Can you work these out from the model? Positions are in its coordinate system, mm. Coordinates: 2 decimals unless noted, no trailing zeros. Order: outer loops, then holes, each group sorted by start corner. A loop starts at its lowest first (then second) coordinate and runs counter-clockwise, first axis right, second up. Notation, with made-up numbers: M -25,65.25 L 28,65.25 A26 ccw 28,85.25 Z; hole C 21,84 d11. An arc over 180 degrees is marked long. Answer as CSV lines item,"result". Start each with the question number.
1. I need wall thicknesses on line 1 along X through (y, z) = (-0.8, 1.25); line 2 along X through (y, z) = (-2.2, 5); line 3 along Z through (x, y) = (10, -1.6). Which ranges of each line are inside material? Lowest first, please. Write a range as from..to.
2. If we mould it in two halves opening along X, with no side actions, what happens to faces 1 (the face through (-11.633, -1.61, 3.643)), 2 (the face through (0, 0, 3)), 3 (the face through (-14.057, -1.61, 3.131)), 4 (the face through (11.666, -1.61, 3.456))? For each: released by +X, released by -X, zero draft, split by the parting line, or undercut.
3. If we section it at D-D (y = -0.5): List the corners of the cut face in (x, z) for me (3 decimals), plus the area to 3 significant figures.
4. If we section it at B-B (y = -2.6): List the corners of the cut face in (x, z) for me (3 decimals).
5. If we section it at A-A (z = 4): List the corners of the cut face in (x, y) for me (3 decimals), plus the area to 3 significant figures.
6. If we section it at C-C (z = 2.5): List the corners of the cut face in (x, y) for me (3 decimals), plus the area to 3 significant figures.
```python
from build123d import *

# Parameters (mm, degrees)
BOSS_EXTRUDE1_DEPTH = 6.35
SKETCH2_R           = 2.159
CUT_EXTRUDE1_DEPTH  = 5.08


with BuildPart() as part:
    # Sketch1 → Boss-Extrude1 (new body)
    with BuildSketch(Plane.XY):
        Polygon((-14.986, 0), (14.986, 0), (13.152912895, -3.175), (-13.152912895, -3.175), align=None)
    extrude(amount=BOSS_EXTRUDE1_DEPTH)

    # Sketch2 → Cut-Extrude1 (cut)
    with BuildSketch(Plane.XZ.offset(3.175)):
        with Locations(Location((-9.525, 3.175, 0), (0, 0, 270))):
            Circle(SKETCH2_R)
        with Locations(Location((9.525, 3.175, 0), (0, 0, 270))):
            Circle(SKETCH2_R)
    extrude(amount=-CUT_EXTRUDE1_DEPTH, mode=Mode.SUBTRACT)


solid = part.part
```
Solved:
1,line 1,"-14.52..-10.5, -8.55..8.55, 10.5..14.52"
1,line 2,"-13.72..-10.68, -8.37..8.37, 10.68..13.72"
1,line 3,"0..1.07, 5.28..6.35"
2,face 1,"undercut"
2,face 2,"zero draft"
2,face 3,"released by -X"
2,face 4,"undercut"
3,outline,"M -14.697,0 L 14.697,0 L 14.697,6.35 L -14.697,6.35 Z; hole C -9.525,3.175 d4.318; hole C 9.525,3.175 d4.318"
3,area,"157 mm²"
4,outline,"M -13.485,0 L 13.485,0 L 13.485,6.35 L -13.485,6.35 Z; hole C -9.525,3.175 d4.318; hole C 9.525,3.175 d4.318"
5,outline,"M -14.986,0 L -13.153,-3.175 L -11.52,-3.175 L -11.52,0 Z; M -7.53,-3.175 L 7.53,-3.175 L 7.53,0 L -7.53,0 Z; M 11.52,-3.175 L 13.153,-3.175 L 14.986,0 L 11.52,0 Z"
5,area,"64.0 mm²"
6,outline,"M -14.986,0 L -13.153,-3.175 L -11.576,-3.175 L -11.576,0 Z; M -7.474,-3.175 L 7.474,-3.175 L 7.474,0 L -7.474,0 Z; M 11.576,-3.175 L 13.153,-3.175 L 14.986,0 L 11.576,0 Z"
6,area,"63.3 mm²"
